Source: CAD feature listing. Evaluate the final solid. Frame: model axes, mm. Give positions to 0.01 mm unless a question says otherwise; leave off trailing zeros. Order: outer loops, then holes, each group sorted by start corner. A loop starts at its lowest first (then second) coordinate and runs counter-clockwise, first axis right, second up.
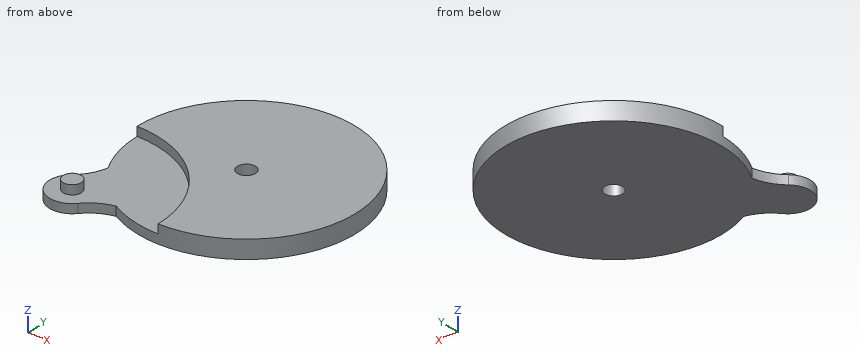
from build123d import *

# Parameters (mm, degrees)
SKICA1_R                 = 60
SKICA1_R_2               = 5
P_IDAT_VYSUNUT_M1_DEPTH  = 10
ODEBRAT_VYSUNUT_M1_DEPTH = 5
P_IDAT_VYSUNUT_M2_DEPTH  = 5
SKICA5_R                 = 5
P_IDAT_VYSUNUT_M3_DEPTH  = 5


with BuildPart() as part:
    # Skica1 → Přidat vysunutím1 (new body)
    with BuildSketch(Plane.XY):
        Circle(SKICA1_R)
        Circle(SKICA1_R_2, mode=Mode.SUBTRACT)
    extrude(amount=P_IDAT_VYSUNUT_M1_DEPTH)

    # Skica2 → Odebrat vysunutím1 (cut)
    with BuildSketch(Plane.XY.offset(10)):
        with BuildLine():
            Line((-60, 0), (-60, -60))
            Line((-60, -60), (0, -60))
            ThreePointArc((0, -60), (-17.573593129, -17.573593129), (-60, 0))
        make_face()
    extrude(amount=-ODEBRAT_VYSUNUT_M1_DEPTH, mode=Mode.SUBTRACT)

    # Skica4 → Přidat vysunutím2 (add)
    with BuildSketch(Plane(origin=(0, 0, 0), x_dir=(-1, 0, 0), z_dir=(0, 0, -1))):
        with BuildLine():
            ThreePointArc((29.001731724, -52.525227815), (42.426406871, -42.426406871), (52.525227815, -29.001731724))
            ThreePointArc((52.525227815, -29.001731724), (55.503659439, -36.872652673), (60.925083435, -43.309314338))
            ThreePointArc((60.925083435, -43.309314338), (61.695066659, -61.695066659), (43.309314338, -60.925083435))
            ThreePointArc((43.309314338, -60.925083435), (36.872652673, -55.503659439), (29.001731724, -52.525227815))
        make_face()
    extrude(amount=-P_IDAT_VYSUNUT_M2_DEPTH)

    # Skica5 → Přidat vysunutím3 (add)
    with BuildSketch(Plane.XY.offset(5)):
        with Locations(Location((-52.856231894, -52.856231894, 0), (0, 0, 180))):
            Circle(SKICA5_R)
    extrude(amount=P_IDAT_VYSUNUT_M3_DEPTH)


solid = part.part
(1) Section B-B, the plane x = -23. Return loops of the section in (y, z).
(2) Line query: line 1 along Y through (x, z) = (0, 3.25); line 2 along Z through (x, y) = (-42, -28); line 3 along Y through (x, z) = (-3.5, 4.25). Output: solid intervals per line, ascending.
(3) Section D-D, the plane x = 32. Return loops of the section in (y, z).
(4) Pin query (flat end, axial travel): pin 1 Ø1 at (y, z) = (-34, 7) entering from +X; pin 2 Ø6 at (y, z) = (-5.5, 5) entering from +X; pin 3 Ø4 at (y, z) = (45.5, 7.5) entering from -X. Return the tip coordinate at first contact, or that it passes through.
(5) Section C-C, the plane y = -46. Return loops of the section in (x, z), plus the area to 3 significant figures.
(6) Section A-A, the plane z = 6.5. Return loops of the section in (x, y), plus the area to 3 significant figures.
Checks:
1. outline: (-55.42, 0) - (55.42, 0) - (55.42, 10) - (-12.77, 10) - (-12.77, 5) - (-55.42, 5) - close
2. line 1: y = -60 to -5, 5 to 60
2. line 2: z = 0 to 5
2. line 3: y = -59.9 to -3.57, 3.57 to 59.9
3. outline: (-50.75, 0) - (50.75, 0) - (50.75, 10) - (-50.75, 10) - close
4. pin 1: stops at x = 49.78
4. pin 2: stops at x = 59.95
4. pin 3: stops at x = -41.32
5. outline: (-63.31, 0) - (38.52, 0) - (38.52, 10) - (-1.66, 10) - (-1.66, 5) - (-63.31, 5) - close
5. area: 710 mm2
6. outline: (-60, 0) arc R60 cw to (0, -60) arc R60 ccw (long way) to start; circle Ø10 at (-52.86, -52.86); hole circle Ø10 at (0, 0)
6. area: 9,250 mm2
